Geometry check sheet. Reference: drawing and pictorial views, mm from the part's lowest x, y, z. A direction names the side the tool comes from. Round coordinates to 2 decimals unless told otherwise and drop trailing zeros. Order: outer loops, then holes, each group sorted by start corner. A loop starts at its lowest first (then second) coordinate and runs counter-clockwise, first axis right, second up. Notation, with made-up numbers: (4.25, 14.25) -> (50.25, 14.25) arc R14 cw to (50.25, 39.25) -> close; hole circle Ø2 at (-40, 68.5). An arc over 180 degrees is marked (long way). Return JSON: item names as keys, results as strings. Group by question number.
1) Draft check along Y on the marked faces 1, 2 and 3. Enter one of: pulls with the +Y half, pulls with the -Y half, needs draft (parallel to the pull), parting line crosses it, or undercut.
2) Tool access check on the marked faces 4, 5 and 6. Record the directions out of +Z, -Z, +X, -X, +Y, -Y that give a thin tool (end or side, any length) a straight path to the whole face; none if there is none.
3) Depth check by flat-ended pin: pin 1 (4 mm diameter, centred on y = 5, z = 47, fed in from +X); pin 2 (3 mm diameter, centred on x = 53, y = 3, fed in from +Z) (1 decimal); pin 3 (4 mm diameter, centred on x = 10.5, y = 4.5, fed in from +Z); pin 4 (6 mm diameter, centred on x = 37.5, y = 3, fed in from -Z). Enter the tip coordinate at first touch or a pass-through.
4) Section check D-D on x = 36. Enter the section's corners in (y, z), plus the area to 3 significant figures.
5) Section check C-C on x = 7.5. Enter the section's corners in (y, z).
6) Section check B-B on y = 5. State how many separate pieces and enclosed holes the cut face has, plus the area to 3 significant figures.
7) Scan lines: L1, parallel to X at y = 5, z = 3.95; L2, parallel to Z at x = 28.75, y = 5; L3, parallel to X at y = 3.5, z = 10. Record each from-to range of solid material in increasing order.
8) Section check A-A on z = 47. Enter the section's corners in (x, y), plus the area to 3 significant figures.
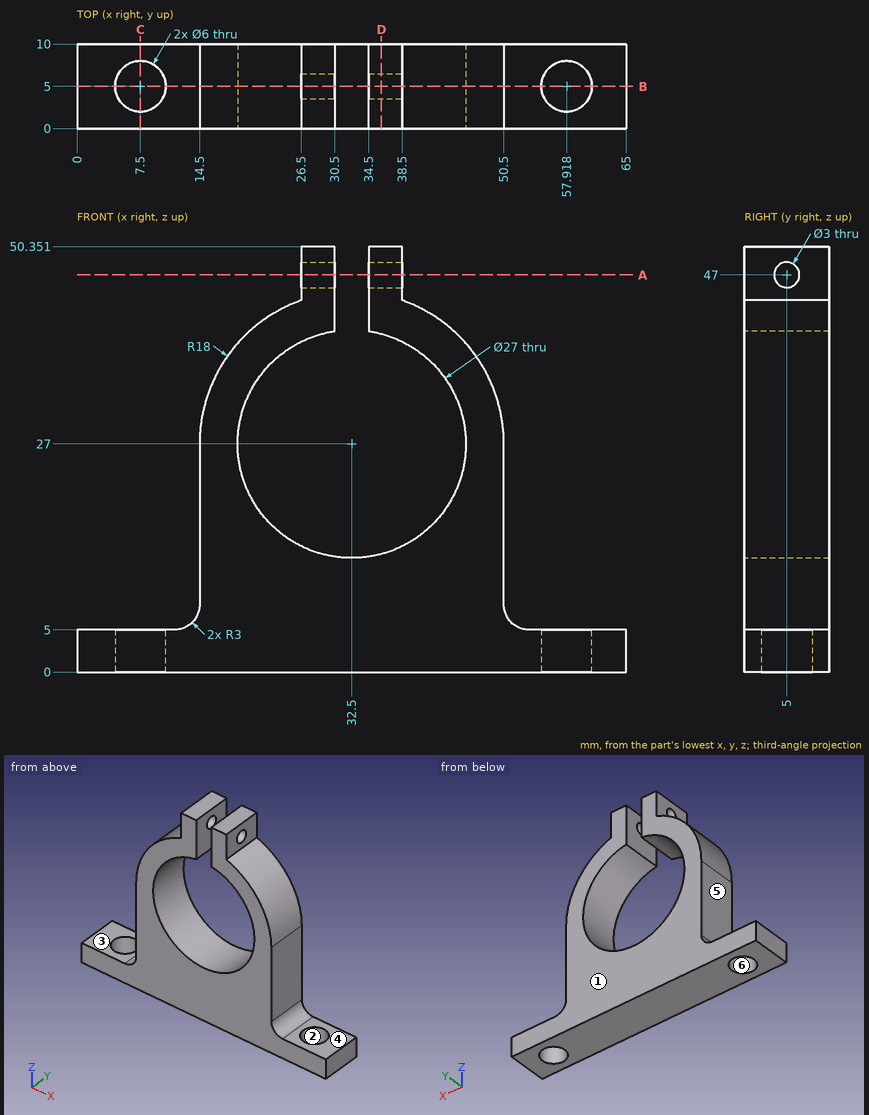
Check result:
{
 "1": {"face 1": "pulls with the +Y half", "face 2": "undercut", "face 3": "needs draft"},
 "2": {"face 4": "+Z, +X, +Y, -Y", "face 5": "+Z, -X, +Y, -Y", "face 6": "+Z, -Z"},
 "3": {"pin 1": "x = 38.5", "pin 2": "z = 5.8", "pin 3": "z = 5.17", "pin 4": "z = 0"},
 "4": {"outline": "(0, 0) -> (10, 0) -> (10, 13.96) -> (0, 13.96) -> close; (0, 40.04) -> (10, 40.04) -> (10, 50.35) -> (0, 50.35) -> close; hole circle Ø3 at (5, 47)", "area": "236 mm^2"},
 "5": {"outline": "(0, 0) -> (2, 0) -> (2, 5) -> (0, 5) -> close; (8, 0) -> (10, 0) -> (10, 5) -> (8, 5) -> close"},
 "6": {"separate pieces": "5", "enclosed holes": "0", "area": "1,000 mm^2"},
 "7": {"L1": "0 to 4.5, 10.5 to 54.92, 60.92 to 65", "L2": "0 to 14.03, 39.97 to 45.5, 48.5 to 50.35", "L3": "14.5 to 50.5"},
 "8": {"outline": "(26.5, 0) -> (30.5, 0) -> (30.5, 3.5) -> (26.5, 3.5) -> close; (26.5, 6.5) -> (30.5, 6.5) -> (30.5, 10) -> (26.5, 10) -> close; (34.5, 0) -> (38.5, 0) -> (38.5, 3.5) -> (34.5, 3.5) -> close; (34.5, 6.5) -> (38.5, 6.5) -> (38.5, 10) -> (34.5, 10) -> close", "area": "56.0 mm^2"}
}
